Could you check a few things on this model? Use its own coordinates, in mm. Face numbers are marked on the shaded views. A direction names the side the tool comes from. Coordinates: 2 decimals unless noted, no trailing zeros. Loops run counter-clockwise (first coordinate to the right, second up) from the corner with the lowest first, then second, coordinate; pieces in that order, holes last.
from build123d import *

# Parameters (mm, degrees)
SKETCH1_W          = 50
SKETCH1_H          = 25
BASE_FLANGE1_DEPTH = 1.5
EDGE_FLANGE1_DEPTH = 25
FILLET1_R          = 12.5
CUT_EXTRUDE1_REACH = 61.245
SKETCH11_R         = 3.75
SKETCH11_R_2       = 1.65
CUT_EXTRUDE2_START = -1.5
SKETCH14_R         = 1.524
CUT_EXTRUDE2_DEPTH = 26.5


# Sheet-metal steps are written as plain solids
with BuildPart() as part:
    # Sketch1 → Base-Flange1 (new body)
    with BuildSketch(Plane(origin=(0, 0, 0), x_dir=(1, 0, 0), z_dir=(0, 1, 0))):
        Rectangle(SKETCH1_W, SKETCH1_H)
    extrude(amount=-BASE_FLANGE1_DEPTH)

    # Edge-Flange1 section (across the edge) → Edge-Flange1 (add)
    with BuildSketch(Plane(origin=(-25.7366, 0, -12.5), x_dir=(1, 0, 0), z_dir=(0, 0, 1))):
        with BuildLine():
            Line((-1.5, 0.7366), (-1.5, 25))
            Line((-1.5, 25), (0, 25))
            Line((0, 25), (0, 0.7366))
            ThreePointArc((0, 0.7366), (0.215745145, 0.215745145), (0.7366, 0))
            Line((0.7366, 0), (0.7366, -1.5))
            ThreePointArc((0.7366, -1.5), (-0.844915027, -0.844915027), (-1.5, 0.7366))
        make_face()
    extrude(amount=EDGE_FLANGE1_DEPTH)

    # Fillet1
    fillet1_edges = [part.edges().sort_by_distance(p)[0] for p in [
        (-26.4866, 25, -12.5),
        (-26.4866, 25, 12.5),
    ]]
    fillet(fillet1_edges, radius=FILLET1_R - 0.0001)  # a hair under: the kernel refuses the full size

    # Sketch11 → Cut-Extrude1 (cut, up to next)
    with BuildSketch(Plane.ZY.offset(27.2366), mode=Mode.PRIVATE) as cut_extrude1_sk1:
        with Locations(Location((0, 12.5, 0), (0, 0, 270))):
            Circle(SKETCH11_R)
    cut_extrude1_tool1 = extrude(cut_extrude1_sk1.sketch, amount=-CUT_EXTRUDE1_REACH, mode=Mode.PRIVATE) & part.part
    # Sketch11 → Cut-Extrude1 (cut, up to next)
    with BuildSketch(Plane.ZY.offset(27.2366), mode=Mode.PRIVATE) as cut_extrude1_sk2:
        with Locations(Location((0, 21, 0), (0, 0, 270))):
            Circle(SKETCH11_R_2)
    cut_extrude1_tool2 = extrude(cut_extrude1_sk2.sketch, amount=-CUT_EXTRUDE1_REACH, mode=Mode.PRIVATE) & part.part
    # Sketch11 → Cut-Extrude1 (cut, up to next)
    with BuildSketch(Plane.ZY.offset(27.2366), mode=Mode.PRIVATE) as cut_extrude1_sk3:
        with Locations(Location((8.5, 12.5, 0), (0, 0, 270))):
            Circle(SKETCH11_R_2)
    cut_extrude1_tool3 = extrude(cut_extrude1_sk3.sketch, amount=-CUT_EXTRUDE1_REACH, mode=Mode.PRIVATE) & part.part
    # Sketch11 → Cut-Extrude1 (cut, up to next)
    with BuildSketch(Plane.ZY.offset(27.2366), mode=Mode.PRIVATE) as cut_extrude1_sk4:
        with Locations(Location((0, 4, 0), (0, 0, 270))):
            Circle(SKETCH11_R_2)
    cut_extrude1_tool4 = extrude(cut_extrude1_sk4.sketch, amount=-CUT_EXTRUDE1_REACH, mode=Mode.PRIVATE) & part.part
    # Sketch11 → Cut-Extrude1 (cut, up to next)
    with BuildSketch(Plane.ZY.offset(27.2366), mode=Mode.PRIVATE) as cut_extrude1_sk5:
        with Locations(Location((-8.5, 12.5, 0), (0, 0, 270))):
            Circle(SKETCH11_R_2)
    cut_extrude1_tool5 = extrude(cut_extrude1_sk5.sketch, amount=-CUT_EXTRUDE1_REACH, mode=Mode.PRIVATE) & part.part
    add(cut_extrude1_tool1.solids().sort_by_distance((-27.2366, 12.5, 0))[0], mode=Mode.SUBTRACT)
    add(cut_extrude1_tool2.solids().sort_by_distance((-27.2366, 21, 0))[0], mode=Mode.SUBTRACT)
    add(cut_extrude1_tool3.solids().sort_by_distance((-27.2366, 12.5, 8.5))[0], mode=Mode.SUBTRACT)
    add(cut_extrude1_tool4.solids().sort_by_distance((-27.2366, 4, 0))[0], mode=Mode.SUBTRACT)
    add(cut_extrude1_tool5.solids().sort_by_distance((-27.2366, 12.5, -8.5))[0], mode=Mode.SUBTRACT)

    # Sketch14 → Cut-Extrude2 (cut)
    with BuildSketch(Plane(origin=(0, 0, 0), x_dir=(1, 0, 0), z_dir=(0, 1, 0)).offset(CUT_EXTRUDE2_START)):
        with Locations(Location((-19.3866, 0, 0), (0, 0, 270))):
            Circle(SKETCH14_R)
        with Locations(Location((-13.0366, 0, 0), (0, 0, 270))):
            Circle(SKETCH14_R)
        with Locations(Location((-6.6866, 0, 0), (0, 0, 270))):
            Circle(SKETCH14_R)
        with Locations(Location((-0.3366, 0, 0), (0, 0, 270))):
            Circle(SKETCH14_R)
        with Locations(Location((6.0134, 0, 0), (0, 0, 270))):
            Circle(SKETCH14_R)
        with Locations(Location((12.3634, 0, 0), (0, 0, 270))):
            Circle(SKETCH14_R)
        with Locations(Location((18.7134, 0, 0), (0, 0, 270))):
            Circle(SKETCH14_R)
        with BuildLine():
            Line((-20.8866, 11.049), (-20.8866, 11.4346))
            ThreePointArc((-20.8866, 11.4346), (-20.574551565, 12.187951565), (-19.8212, 12.5))
            Line((-19.8212, 12.5), (-18.65, 12.5))
            ThreePointArc((-18.65, 12.5), (-17.896648435, 12.187951565), (-17.5846, 11.4346))
            Line((-17.5846, 11.4346), (-17.5846, 11.049))
            ThreePointArc((-17.5846, 11.049), (-16.0606, 9.525), (-14.5366, 11.049))
            Line((-14.5366, 11.049), (-14.5366, 11.4346))
            ThreePointArc((-14.5366, 11.4346), (-14.224551565, 12.187951565), (-13.4712, 12.5))
            Line((-13.4712, 12.5), (-12.3, 12.5))
            ThreePointArc((-12.3, 12.5), (-11.546648435, 12.187951565), (-11.2346, 11.4346))
            Line((-11.2346, 11.4346), (-11.2346, 11.049))
            ThreePointArc((-11.2346, 11.049), (-9.7106, 9.525), (-8.1866, 11.049))
            Line((-8.1866, 11.049), (-8.1866, 11.4346))
            ThreePointArc((-8.1866, 11.4346), (-7.874551565, 12.187951565), (-7.1212, 12.5))
            Line((-7.1212, 12.5), (-5.95, 12.5))
            ThreePointArc((-5.95, 12.5), (-5.196648435, 12.187951565), (-4.8846, 11.4346))
            Line((-4.8846, 11.4346), (-4.8846, 11.049))
            ThreePointArc((-4.8846, 11.049), (-3.3606, 9.525), (-1.8366, 11.049))
            Line((-1.8366, 11.049), (-1.8366, 11.4346))
            ThreePointArc((-1.8366, 11.4346), (-1.524551565, 12.187951565), (-0.7712, 12.5))
            Line((-0.7712, 12.5), (0.4, 12.5))
            ThreePointArc((0.4, 12.5), (1.153351565, 12.187951565), (1.4654, 11.4346))
            Line((1.4654, 11.4346), (1.4654, 11.049))
            ThreePointArc((1.4654, 11.049), (2.9894, 9.525), (4.5134, 11.049))
            Line((4.5134, 11.049), (4.5134, 11.4346))
            ThreePointArc((4.5134, 11.4346), (4.825448435, 12.187951565), (5.5788, 12.5))
            Line((5.5788, 12.5), (6.75, 12.5))
            ThreePointArc((6.75, 12.5), (7.503351565, 12.187951565), (7.8154, 11.4346))
            Line((7.8154, 11.4346), (7.8154, 11.049))
            ThreePointArc((7.8154, 11.049), (9.3394, 9.525), (10.8634, 11.049))
            Line((10.8634, 11.049), (10.8634, 11.4346))
            ThreePointArc((10.8634, 11.4346), (11.175448435, 12.187951565), (11.9288, 12.5))
            Line((11.9288, 12.5), (13.1, 12.5))
            ThreePointArc((13.1, 12.5), (13.853351565, 12.187951565), (14.1654, 11.4346))
            Line((14.1654, 11.4346), (14.1654, 11.049))
            ThreePointArc((14.1654, 11.049), (15.6894, 9.525), (17.2134, 11.049))
            Line((17.2134, 11.049), (17.2134, 11.4346))
            ThreePointArc((17.2134, 11.4346), (17.525448435, 12.187951565), (18.2788, 12.5))
            ThreePointArc((18.2788, 12.5), (23.031406098, 10.531406098), (25, 5.7788))
            Line((25, 5.7788), (25, 3.086206539))
            Line((25, 3.086206539), (30.090944924, 3.086206539))
            Line((30.090944924, 3.086206539), (30.090944924, 14.304286601))
            Line((30.090944924, 14.304286601), (18.2788, 14.304286601))
            Line((18.2788, 14.304286601), (-25, 14.304286601))
            Line((-25, 14.304286601), (-25, 12.5))
            ThreePointArc((-25, 12.5), (-24.246648435, 12.187951565), (-23.9346, 11.4346))
            Line((-23.9346, 11.4346), (-23.9346, 11.049))
            ThreePointArc((-23.9346, 11.049), (-22.4106, 9.525), (-20.8866, 11.049))
        make_face()
        with BuildLine():
            Line((30.090944924, -14.304286601), (18.2788, -14.304286601))
            Line((18.2788, -14.304286601), (-25, -14.304286601))
            Line((-25, -14.304286601), (-25, -12.5))
            ThreePointArc((-25, -12.5), (-24.246648435, -12.187951565), (-23.9346, -11.4346))
            Line((-23.9346, -11.4346), (-23.9346, -11.049))
            ThreePointArc((-23.9346, -11.049), (-22.4106, -9.525), (-20.8866, -11.049))
            Line((-20.8866, -11.049), (-20.8866, -11.4346))
            ThreePointArc((-20.8866, -11.4346), (-20.574551565, -12.187951565), (-19.8212, -12.5))
            Line((-19.8212, -12.5), (-18.65, -12.5))
            ThreePointArc((-18.65, -12.5), (-17.896648435, -12.187951565), (-17.5846, -11.4346))
            Line((-17.5846, -11.4346), (-17.5846, -11.049))
            ThreePointArc((-17.5846, -11.049), (-16.0606, -9.525), (-14.5366, -11.049))
            Line((-14.5366, -11.049), (-14.5366, -11.4346))
            ThreePointArc((-14.5366, -11.4346), (-14.224551565, -12.187951565), (-13.4712, -12.5))
            Line((-13.4712, -12.5), (-12.3, -12.5))
            ThreePointArc((-12.3, -12.5), (-11.546648435, -12.187951565), (-11.2346, -11.4346))
            Line((-11.2346, -11.4346), (-11.2346, -11.049))
            ThreePointArc((-11.2346, -11.049), (-9.7106, -9.525), (-8.1866, -11.049))
            Line((-8.1866, -11.049), (-8.1866, -11.4346))
            ThreePointArc((-8.1866, -11.4346), (-7.874551565, -12.187951565), (-7.1212, -12.5))
            Line((-7.1212, -12.5), (-5.95, -12.5))
            ThreePointArc((-5.95, -12.5), (-5.196648435, -12.187951565), (-4.8846, -11.4346))
            Line((-4.8846, -11.4346), (-4.8846, -11.049))
            ThreePointArc((-4.8846, -11.049), (-3.3606, -9.525), (-1.8366, -11.049))
            Line((-1.8366, -11.049), (-1.8366, -11.4346))
            ThreePointArc((-1.8366, -11.4346), (-1.524551565, -12.187951565), (-0.7712, -12.5))
            Line((-0.7712, -12.5), (0.4, -12.5))
            ThreePointArc((0.4, -12.5), (1.153351565, -12.187951565), (1.4654, -11.4346))
            Line((1.4654, -11.4346), (1.4654, -11.049))
            ThreePointArc((1.4654, -11.049), (2.9894, -9.525), (4.5134, -11.049))
            Line((4.5134, -11.049), (4.5134, -11.4346))
            ThreePointArc((4.5134, -11.4346), (4.825448435, -12.187951565), (5.5788, -12.5))
            Line((5.5788, -12.5), (6.75, -12.5))
            ThreePointArc((6.75, -12.5), (7.503351565, -12.187951565), (7.8154, -11.4346))
            Line((7.8154, -11.4346), (7.8154, -11.049))
            ThreePointArc((7.8154, -11.049), (9.3394, -9.525), (10.8634, -11.049))
            Line((10.8634, -11.049), (10.8634, -11.4346))
            ThreePointArc((10.8634, -11.4346), (11.175448435, -12.187951565), (11.9288, -12.5))
            Line((11.9288, -12.5), (13.1, -12.5))
            ThreePointArc((13.1, -12.5), (13.853351565, -12.187951565), (14.1654, -11.4346))
            Line((14.1654, -11.4346), (14.1654, -11.049))
            ThreePointArc((14.1654, -11.049), (15.6894, -9.525), (17.2134, -11.049))
            Line((17.2134, -11.049), (17.2134, -11.4346))
            ThreePointArc((17.2134, -11.4346), (17.525448435, -12.187951565), (18.2788, -12.5))
            ThreePointArc((18.2788, -12.5), (23.031406098, -10.531406098), (25, -5.7788))
            Line((25, -5.7788), (25, -3.086206539))
            Line((25, -3.086206539), (30.090944924, -3.086206539))
            Line((30.090944924, -3.086206539), (30.090944924, -14.304286601))
        make_face()
    extrude(amount=CUT_EXTRUDE2_DEPTH, mode=Mode.SUBTRACT)


solid = part.part
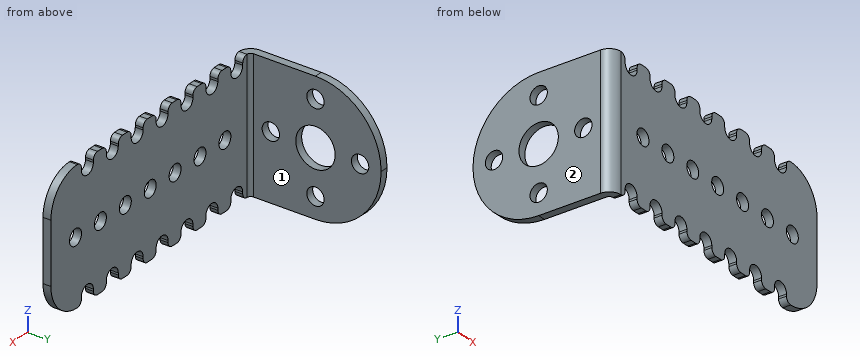
(1) Which directions (+Z, -Z, +X, -X, +Y, -Y) give clear straight access to the entire face, cutting with the end or side of a thin tool? Please do the marked faces 1 and 2.
Answers:
face 1: +Z, -Z, +X, +Y
face 2: +Z, -Z, -X, +Y, -Y
(2) Imagine slicing it at D-D, the plane y = 7. Write out the boundary of the cut face in (x, z).
Answers:
outline: (-27.24, -12.5) - (-25.74, -12.5) - (-25.74, 12.5) - (-27.24, 12.5) - close
(3) Imagine slicing it at A-A, the plane z = -2.25. Write out the boundary of the cut face in (x, y), and give its area (3 significant figures).
Answers:
outline: (-27.24, 0.74) arc R2.24 ccw to (-25, -1.5) - (25, -1.5) - (25, 0) - (-25, 0) arc R0.74 cw to (-25.74, 0.74) - (-25.74, 9.5) - (-27.24, 9.5) - close; (-27.24, 15.5) - (-25.74, 15.5) - (-25.74, 24.8) - (-27.24, 24.8) - close
area: 106 mm2
(4) Imagine slicing it at B-B, the plane y = 4. Write out the boundary of the cut face in (x, z), and give its area (4 significant figures).
Answers:
outline: (-27.24, -12.5) - (-25.74, -12.5) - (-25.74, -1.65) - (-27.24, -1.65) - close; (-27.24, 1.65) - (-25.74, 1.65) - (-25.74, 12.5) - (-27.24, 12.5) - close
area: 32.55 mm2
(5) For pin 1 (8 mm diameter, centred on x = 5, y = 7.5, fed in from -Z); pin 2 (6 mm diameter, centred on y = 13, z = -4.5, fed in from +X); pin 3 (3 mm diameter, centred on x = 14.5, z = -3.5, fed in from +Y), each with a flat end and sliding along its axis, tell me the tip position at first contact or that it passes through.
Answers:
pin 1: passes through
pin 2: stops at x = -25.74
pin 3: stops at y = 0
(6) I need wall thicknesses on probe 1 along Y at (x, z) = (-24, 9); probe 2 along X at (y, z) = (18.25, -6). Which ranges of each line are inside material? Lowest first, please.
Answers:
probe 1: y = -1.5 to 0
probe 2: x = -27.24 to -25.74
(7) Imagine slicing it at C-C, the plane z = 5. Write out the boundary of the cut face in (x, y), and give its area (3 significant figures).
Answers:
outline: (-27.24, 0.74) arc R2.24 ccw to (-25, -1.5) - (25, -1.5) - (25, 0) - (-25, 0) arc R0.74 cw to (-25.74, 0.74) - (-25.74, 23.96) - (-27.24, 23.96) - close
area: 113 mm2
